```python
from build123d import *

# Parameters (mm, degrees)
BOSS_EXTRUDE1_DEPTH = 57.15
SKETCH2_R           = 3.2639
CUT_EXTRUDE1_DEPTH  = 12.7


with BuildPart() as part:
    # Sketch1 → Boss-Extrude1 (new body, symmetric)
    with BuildSketch(Plane(origin=(0, 0, 0), x_dir=(1, 0, 0), z_dir=(0, 1, 0))):
        Polygon((6.434399754, 3.515939866), (0.172306635, 7.330323578), (-6.262093119, 3.814383712), (-6.434399754, -3.515939866), (-0.172306635, -7.330323578), (6.262093119, -3.814383712), align=None)
    extrude(amount=BOSS_EXTRUDE1_DEPTH, both=True)

    # Sketch2 → Cut-Extrude1 (cut)
    with BuildSketch(Plane(origin=(0, 57.15, 0), x_dir=(1, 0, 0), z_dir=(0, 1, 0))):
        Circle(SKETCH2_R)
    cut_extrude1 = extrude(amount=-CUT_EXTRUDE1_DEPTH, mode=Mode.SUBTRACT)

    # Mirror1: Cut-Extrude1 across plane
    add(cut_extrude1.mirror(Plane.ZX), mode=Mode.SUBTRACT)


solid = part.part
```
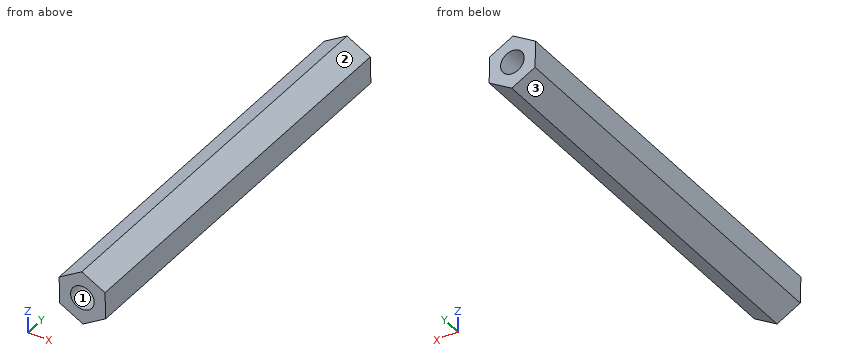
Work out the finished part from the listing and answer in its coordinate system (mm). Face numbers are marked on the shaded views. Give positions to 0.01 mm unless a question says otherwise; leave off trailing zeros. Order: outer loops, then holes, each group sorted by start corner. A loop starts at its lowest first (then second) coordinate and runs counter-clockwise, first axis right, second up. Notation, with made-up numbers: (49, 3) - (60, 3) arc R6 ccw to (60, 10) - close; hole circle Ø10 at (71.25, 30). An arc over 180 degrees is marked (long way). One line per item, written item: value. Start each with the question number.
1. Section C-C, the plane x = -1.25 is taken. Write down the section's boundary in (y, z), then the cut area to 3 significant figures.
2. Section B-B, the plane y = -20 is taken. Write down the section's boundary in (x, z), then the cut area to 3 significant figures.
3. Each of these flat-tipped pins is pushed along its axis until it touches: pin 1 Ø3.5 at (x, z) = (-1.5, 0.5) entering from -Y; pin 2 Ø6 at (x, z) = (0, 0) entering from +Y; pin 3 Ø6 at (y, z) = (36, -4) entering from -X; pin 4 Ø1.5 at (y, z) = (-19, -1) entering from +X. Where does it stop, or does it pass through?
4. Consider line 1 (X direction, y = -44, z = -3); line 2 (Y direction, x = -2, z = -0.5); line 3 (X direction, y = -50, z = 0). Determine where each line is inside the solid, lowest interval first.
5. Section D-D, the plane z = -2 is taken. Write down the section's boundary in (x, y).
6. Section A-A, the plane y = -46.5 is taken. Write down the section's boundary in (x, z), then the cut area to 3 significant figures.
7. For a pull along Z with two mould halves and no side action, classify the marked faces 1, 2 and 3 as released by +Z, released by -Z, zero draft, split by the parting line, or undercut.
Filled sheet:
1. outline: (-57.15, -6.55) - (57.15, -6.55) - (57.15, -3.02) - (44.45, -3.02) - (44.45, 3.02) - (57.15, 3.02) - (57.15, 6.67) - (-57.15, 6.67) - (-57.15, 3.02) - (-44.45, 3.02) - (-44.45, -3.02) - (-57.15, -3.02) - close
1. area: 1,360 mm²
2. outline: (-6.43, 3.52) - (-6.26, -3.81) - (0.17, -7.33) - (6.43, -3.52) - (6.26, 3.81) - (-0.17, 7.33) - close
2. area: 140 mm²
3. pin 1: y = -57.15
3. pin 2: y = 44.45
3. pin 3: x = -6.33
3. pin 4: x = 6.39
4. line 1: -6.28 to 6.42
4. line 2: -44.45 to 44.45
4. line 3: -6.35 to -3.26, 3.26 to 6.35
5. outline: (-6.3, -57.15) - (-2.58, -57.15) - (-2.58, -44.45) - (2.58, -44.45) - (2.58, -57.15) - (6.4, -57.15) - (6.4, 57.15) - (2.58, 57.15) - (2.58, 44.45) - (-2.58, 44.45) - (-2.58, 57.15) - (-6.3, 57.15) - close
6. outline: (-6.43, 3.52) - (-6.26, -3.81) - (0.17, -7.33) - (6.43, -3.52) - (6.26, 3.81) - (-0.17, 7.33) - close; hole circle Ø6.53 at (0, 0)
6. area: 106 mm²
7. face 1: undercut
7. face 2: released by +Z
7. face 3: released by -Z
